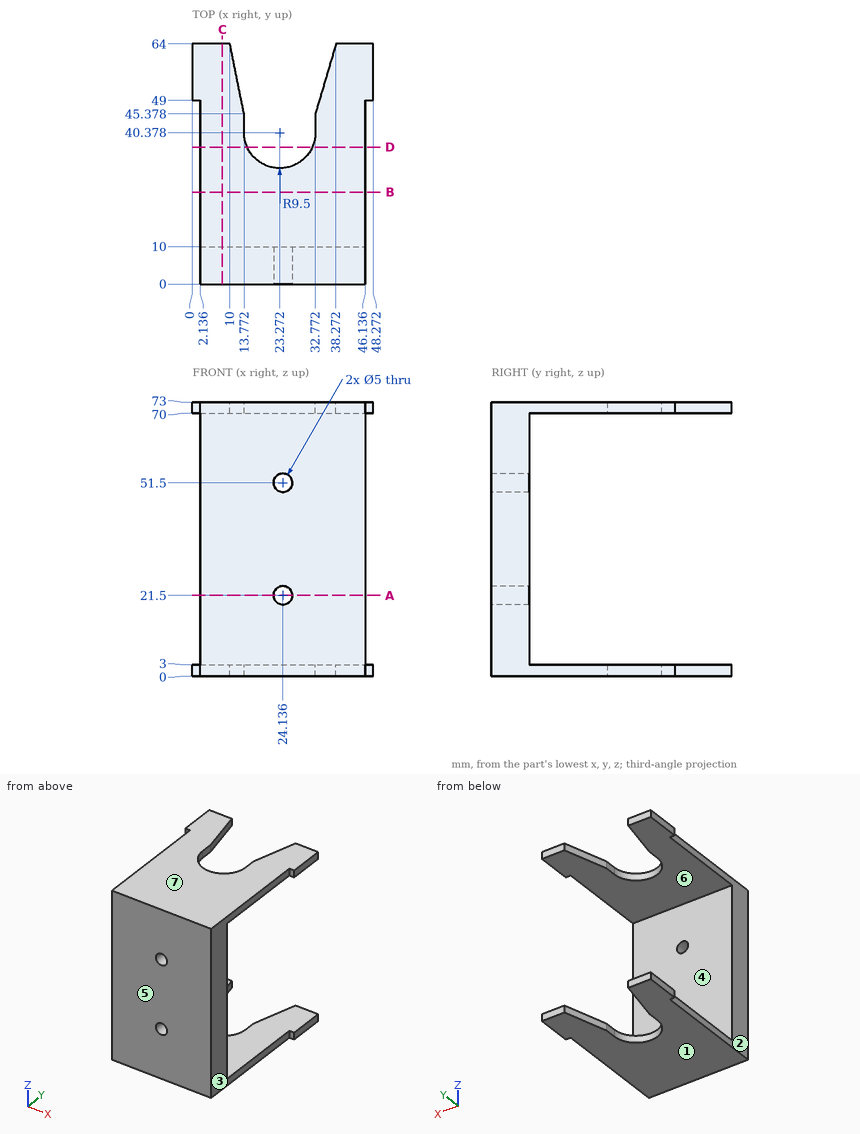
Geometry: see drawing. Coordinates: mm, zero at the bounding-box minimum. A direction names the side the tool comes from. Give positions to 0.01 mm unless a question says otherwise; leave off trailing zeros. Loops run counter-clockwise (first coordinate to the right, second up) from the corner with the lowest first, then second, coordinate; pieces in that order, holes last. Notation, with made-up numbers: (70.5, -17) -> (98.5, -17) arc R11 cw to (98.5, -2) -> close; hole circle Ø3 at (-37.75, -4). An arc over 180 degrees is marked (long way). Put each result on its own line as item: value.
1. Cut plane A-A (z = 21.5). Return the cut outline in (x, y), plus the area to 3 significant figures.
Taken from the geometry:
outline: (2.14, 0) -> (21.64, 0) -> (21.64, 10) -> (2.14, 10) -> close; (26.64, 0) -> (46.14, 0) -> (46.14, 10) -> (26.64, 10) -> close
area: 390 mm2
2. Cut plane B-B (y = 24.5). Return the cut outline in (x, z).
Taken from the geometry:
outline: (2.14, 0) -> (46.14, 0) -> (46.14, 3) -> (2.14, 3) -> close; (2.14, 70) -> (46.14, 70) -> (46.14, 73) -> (2.14, 73) -> close
3. Pin query (flat end, axial travel): P1, Ø13, axis at x = 14, z = 46.5, coming from the +Y side; P2, Ø1.5, axis at y = 44, z = 71.5, coming from the +X side; P3, Ø12, axis at x = 33, y = 31.5, coming from the -Z side; P4, Ø1.1, axis at x = 47, z = 2, coming from the -Y side. Return the tip coordinate at first contact, or that it passes through.
Taken from the geometry:
P1: stops at y = 10
P2: stops at x = 46.14
P3: stops at z = 0
P4: stops at y = 49
4. Cut plane C-C (x = 8). Return the cut outline in (y, z), plus the area to 3 significant figures.
Taken from the geometry:
outline: (0, 0) -> (64, 0) -> (64, 3) -> (10, 3) -> (10, 70) -> (64, 70) -> (64, 73) -> (0, 73) -> close
area: 1,050 mm2
5. Set-up query: the marked faces 1, 2, 3 and 4. Return all of +Z, -Z, +X, -X, +Y, -Y with unobstructed straight access to the full face (end or side cutting, diameter ignored); none if empty.
Taken from the geometry:
face 1: -Z, +X, -X, +Y, -Y
face 2: +Z, -Z, -X, -Y
face 3: +Z, -Z, +X, -Y
face 4: +X, -X, +Y
6. Ray query, line 1 along X through (y, z) = (7.75, 51.5); line 2 along Z through (x, y) = (7, 58.5); line 3 along Z through (x, y) = (23.5, 3). Return the intervals inside material, ascending. Write a range as [from, to].
Taken from the geometry:
line 1: x = [2.14, 21.64], [26.64, 46.14]
line 2: z = [0, 3], [70, 73]
line 3: z = [0, 19.08], [23.92, 49.08], [53.92, 73]
7. Cut plane D-D (y = 36.5). Return the cut outline in (x, z) (1 decimal).
Taken from the geometry:
outline: (2.1, 0) -> (14.6, 0) -> (14.6, 3) -> (2.1, 3) -> close; (2.1, 70) -> (14.6, 70) -> (14.6, 73) -> (2.1, 73) -> close; (31.9, 0) -> (46.1, 0) -> (46.1, 3) -> (31.9, 3) -> close; (31.9, 70) -> (46.1, 70) -> (46.1, 73) -> (31.9, 73) -> close
8. Pull-direction query (Z, two-part tool) for the marked faces 5, 6 and 7; classes: released by +Z, released by -Z, zero draft, split by the parting line, or undercut.
Taken from the geometry:
face 5: zero draft
face 6: undercut
face 7: released by +Z
